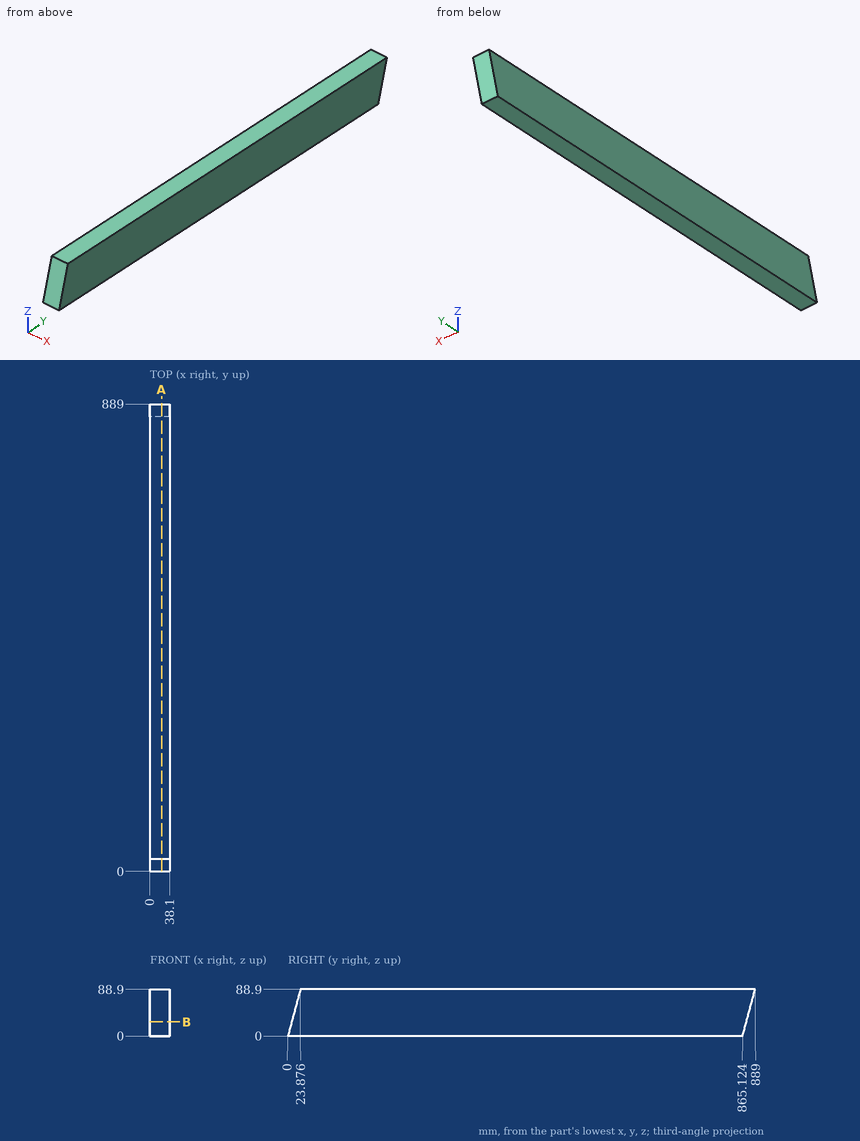
Geometry: see drawing. Coordinates: mm, zero at the bounding-box minimum. Round coordinates to 2 decimals unless told otherwise and drop trailing zeros. Loops run counter-clockwise (first coordinate to the right, second up) from the corner with the lowest first, then second, coordinate; pieces in that order, holes last. Notation, with made-up numbers: M 84.5,23.5 L 134.5,23.5 A14 ccw 134.5,27.5 Z; hole C 53,-22 d1. An arc over 180 degrees is marked long. Use a Markdown table: item, result. Add a question column.
1. Cut plane A-A, the plane x = 22.5. Output: boundary loops of the cut face in (y, z).
2. Ray query, line 1 along Y through (x, z) = (36, 59.5); line 2 along Y through (x, z) = (28, 71). Return the intervals inside material, ascending. Write a range as [from, to].
3. Cut plane B-B, the plane z = 27. Output: boundary loops of the cut face in (x, y).
4. Contact query for flat-ended pins moving along their axis: pin 1 (6 mm diameter, centred on x = 4.5, z = 34, fed in from +Y); pin 2 (12 mm diameter, centred on x = 15.5, z = 53.5, fed in from +Y); pin 3 (1 mm diameter, centred on x = 31.5, z = 67.5, fed in from +Y). Output: stop coordinate, or through.
Solution:
| question | item | result |
|---|---|---|
| 1 | outline | M 0,0 L 865.12,0 L 889,88.9 L 23.88,88.9 Z |
| 2 | line 1 | y = [15.98, 881.1] |
| 2 | line 2 | y = [19.07, 884.19] |
| 3 | outline | M 0,7.25 L 38.1,7.25 L 38.1,872.38 L 0,872.38 Z |
| 4 | pin 1 | stops at y = 875.06 |
| 4 | pin 2 | stops at y = 881.1 |
| 4 | pin 3 | stops at y = 883.39 |
